For this review, take the finished solid that the model builds, in its own axes (mm). A direction names the side the tool comes from. Give positions to 0.01 mm unless a question says otherwise; leave off trailing zeros.
Q1. Machinability: for faces 1 (the flat face through (-15.5, 0, 123)), 2 (the flat face through (0, 0, 0)), which of the approach directions +Z, -Z, +X, -X, +Y, -Y give a long, thin tool a straight path to every point of the face, cutting with its end or side? Answer none if there is none.
Q2. For line 1 (X direction, y = -4.75, z = 120), list the stretches that pass through material, from the lowest coordinate up.
Q3. Insertion check: P1, Ø1.6, axis at x = -16.5, y = -5, coming from the +Z side; P2, Ø7.5, axis at y = 5, z = 124, coming from the -X side. Each pin has a flat end and moves straight along its axis. Give the tip position at first contact, or say it passes through.
Autodesk Inventor part; units mm, degrees
ref_plane "YZ Plane" through (0, 0, 0) normal (1, 0, 0) x (0, 1, 0)
ref_plane "XZ Plane" through (0, 0, 0) normal (0, 1, 0) x (-1, 0, 0)
ref_plane "XY Plane" through (0, 0, 0) normal (0, 0, 1) x (1, 0, 0)
sketch "Sketch1" plane through (0, 0, 0) normal (0, 0, 1) x (1, 0, 0)
  line L0 (-17.5, -12.5) -> (17.5, -12.5)
  line L1 (17.5, -12.5) -> (17.5, 12.5)
  line L2 (17.5, 12.5) -> (-17.5, 12.5)
  line L3 (-17.5, 12.5) -> (-17.5, -12.5)
  line L4 (-17.5, -12.5) -> (17.5, 12.5) construction
  line L5 (17.5, -12.5) -> (-17.5, 12.5) construction
  point P0 (0, 0)
  dimension "d0" = 35
  dimension "d1" = 25
extrude "Extrusion1" add sketch "Sketch1" along normal blind 130
sketch "Sketch2" plane through (-17.5, -12.5, 0) normal (0, -1, 0) x (1, 0, 0)
  line L0 (2, 115) -> (0, 115)
  line L1 (0, 115) -> (0, 130)
  line L2 (0, 130) -> (2, 130)
  line L3 (2, 130) -> (2, 115)
  line L4 (0, 0) -> (0, 130)
  line L5 (0, 130) -> (35, 130)
  point P0 (17.5, 0)
  dimension "d4" = 2
  dimension "d5" = 15
extrude "Extrusion2" cut sketch "Sketch2" against normal through all
properties part number "Distanzblock" material "Aluminum 6061"
Computed:
1. face 1: +Z, -X, +Y, -Y
1. face 2: -Z, +X, -X, +Y, -Y
2. line 1: x = -15.5 to 17.5
3. P1: stops at z = 115
3. P2: stops at x = -15.5
